```python
from build123d import *

# Parameters (mm, degrees)
BOSS_EXTRUDE1_DEPTH         = 19.05
SKETCH2_R                   = 3.175
CUT_EXTRUDE1_DEPTH          = 42.790767895
CHAMFER1_SIZE               = 3.175
SKETCH3_R                   = 25.2095
BOSS_EXTRUDE2_DEPTH         = 38.1
CHAMFER2_SIZE               = 0.79375
F_4_40_TAPPED_HOLE1_REACH   = 77.334
F_4_40_TAPPED_HOLE1_BORE_R  = 1.1303
F_3_8_16_TAPPED_HOLE1_D     = 7.9375
F_3_8_16_TAPPED_HOLE1_DEPTH = 25.4
F_3_8_16_TAPPED_HOLE1_TIP   = 2.384665582


with BuildPart() as part:
    # Sketch1 → Boss-Extrude1 (new body)
    with BuildSketch(Plane.XY):
        Polygon((-7.14375, 15.875), (-7.14375, -4.7625), (-14.2875, -4.7625), (-14.2875, 23.8125), (14.2875, 23.8125), (14.2875, -4.7625), (7.14375, -4.7625), (7.14375, 15.875), align=None)
    extrude(amount=BOSS_EXTRUDE1_DEPTH)

    # Sketch2 → Cut-Extrude1 (cut, through all)
    with BuildSketch(Plane(origin=(14.2875, 0, 0), x_dir=(0, 0, -1), z_dir=(1, 0, 0))):
        with Locations((-9.525, 0)):
            Circle(SKETCH2_R)
    extrude(amount=-CUT_EXTRUDE1_DEPTH, mode=Mode.SUBTRACT)

    # Chamfer1
    chamfer1_edges = [part.edges().sort_by_distance(p)[0] for p in [
        (10.715625, -4.7625, 19.05),
        (-10.715625, -4.7625, 19.05),
        (-10.715625, -4.7625, 0),
        (10.715625, -4.7625, 0),
    ]]
    chamfer(chamfer1_edges, length=CHAMFER1_SIZE)

    # Sketch3 → Boss-Extrude2 (add)
    with BuildSketch(Plane(origin=(0, 23.8125, 0), x_dir=(1, 0, 0), z_dir=(0, 1, 0))):
        with Locations(Location((0, -9.525, 0), (0, 0, 90))):
            Circle(SKETCH3_R)
    extrude(amount=BOSS_EXTRUDE2_DEPTH)

    # Chamfer2
    chamfer2_edges = [part.edges().sort_by_distance(p)[0] for p in [
        (0, 23.8125, 34.7345),
        (0, 61.9125, 34.7345),
    ]]
    chamfer(chamfer2_edges, length=CHAMFER2_SIZE)

    # #4-40 Tapped Hole1 bore → #4-40 Tapped Hole1 (cut, up to next)
    with BuildSketch(Plane.XY.offset(19.05), mode=Mode.PRIVATE) as f_4_40_tapped_hole1_sk1:
        with Locations((-10.715625, 0)):
            Circle(F_4_40_TAPPED_HOLE1_BORE_R)
    f_4_40_tapped_hole1_tool1 = extrude(f_4_40_tapped_hole1_sk1.sketch, amount=-F_4_40_TAPPED_HOLE1_REACH, mode=Mode.PRIVATE) & part.part
    # #4-40 Tapped Hole1 bore → #4-40 Tapped Hole1 (cut, up to next)
    with BuildSketch(Plane.XY.offset(19.05), mode=Mode.PRIVATE) as f_4_40_tapped_hole1_sk2:
        with Locations((10.715625, 0)):
            Circle(F_4_40_TAPPED_HOLE1_BORE_R)
    f_4_40_tapped_hole1_tool2 = extrude(f_4_40_tapped_hole1_sk2.sketch, amount=-F_4_40_TAPPED_HOLE1_REACH, mode=Mode.PRIVATE) & part.part
    add(f_4_40_tapped_hole1_tool1.solids().sort_by_distance((-10.715625, 0, 19.05))[0], mode=Mode.SUBTRACT)
    add(f_4_40_tapped_hole1_tool2.solids().sort_by_distance((10.715625, 0, 19.05))[0], mode=Mode.SUBTRACT)

    # 3/8-16 Tapped Hole1
    with Locations(Plane(origin=(25.2095, 0, 0), x_dir=(0, 0, -1), z_dir=(1, 0, 0))):
        with Locations((-9.525, 51.1429)):
            Hole(F_3_8_16_TAPPED_HOLE1_D / 2, depth=F_3_8_16_TAPPED_HOLE1_DEPTH)
            with Locations((0, 0, -(F_3_8_16_TAPPED_HOLE1_DEPTH + F_3_8_16_TAPPED_HOLE1_TIP / 2))):  # 118° drill point
                Cone(0, F_3_8_16_TAPPED_HOLE1_D / 2, F_3_8_16_TAPPED_HOLE1_TIP, mode=Mode.SUBTRACT)


solid = part.part
```
Could you check a few things on this model? Use its own coordinates, in mm. A direction names the side the tool comes from. Round coordinates to 2 decimals unless told otherwise and drop trailing zeros. Loops run counter-clockwise (first coordinate to the right, second up) from the corner with the lowest first, then second, coordinate; pieces in that order, holes last. Notation, with made-up numbers: M 88.25,-15.75 L 121.25,-15.75 A14 cw 121.25,-3.75 Z; hole C 63.25,23 d1. An arc over 180 degrees is marked long. Write item = value, one per line.
1. Which directions (+Z, -Z, +X, -X, +Y, -Y) give clear straight access to the entire face, cutting with the end or side of a thin tool? Please do faces 1 (the face through (0, 17, 0)), 2 (the face through (0, 17, 19.05)), 3 (the face through (10.766, 0.954, 6.497)), 4 (the face through (11.76, -0.43, 15.82)), 5 (the face through (14.288, 10, 9)).
Results below:
face_1 = -Z, +X, -X, -Y
face_2 = +Z, +X, -X, -Y
face_3 = +X, -X
face_4 = +Z
face_5 = +Z, -Z, +X, -Y
2. I want a section at D-D, the plane y = 36. Write out the boundary of the cut face in (x, z) (1 decimal).
Results below:
outline = C 0,9.5 d50.4
3. I need wall thicknesses on probe 1 along X at (y, z) = (0, 17.5); probe 2 along Z at (x, y) = (-9.25, 0); probe 3 along X at (y, z) = (17.5, 15.5). Which ranges of each line are inside material? Lowest first, please.
Results below:
probe_1 = -14.29 to -11.85, -9.59 to -7.14, 7.14 to 9.59, 11.85 to 14.29
probe_2 = 0 to 6.35, 12.7 to 19.05
probe_3 = -14.29 to 14.29
4. I want a section at C-C, the plane x = 8. Count the separate pieces of the cut face and the enclosed holes in it, and give its area (3 significant figures).
Results below:
separate_pieces = 1
enclosed_holes = 2
area = 2,270 mm²
5. I want a section at A-A, the plane y = 9.5. Write out the boundary of the cut face in (x, z).
Results below:
outline = M -14.29,0 L -7.14,0 L -7.14,19.05 L -14.29,19.05 Z; M 7.14,0 L 14.29,0 L 14.29,19.05 L 7.14,19.05 Z
6. I want a section at B-B, the plane y = 0. Write out the boundary of the cut face in (x, z), and give its area (3 significant figures).
Results below:
outline = M -14.29,0 L -7.14,0 L -7.14,6.35 L -14.29,6.35 Z; M -14.29,12.7 L -11.85,12.7 L -11.85,19.05 L -14.29,19.05 Z; M -9.59,12.7 L -7.14,12.7 L -7.14,19.05 L -9.59,19.05 Z; M 7.14,0 L 14.29,0 L 14.29,6.35 L 7.14,6.35 Z; M 7.14,12.7 L 9.59,12.7 L 9.59,19.05 L 7.14,19.05 Z; M 11.85,12.7 L 14.29,12.7 L 14.29,19.05 L 11.85,19.05 Z
area = 153 mm²
7. Thinking about a two-plate mould opening in X: for faces 6 (the face through (-17.038, 42.607, 28.105)), 7 (the face through (-2.16, 51.83, 9.61)), 8 (the face through (7.144, 5, 9)), 9 (the face through (-7.144, 6, 9)), which applies, +X half, -X half, draft (parallel to the pull), parting line (faces both ways), or undercut?
Results below:
face_6 = parting line
face_7 = +X half
face_8 = undercut
face_9 = undercut
8. Will these pins go through, and if not, where does the flat tip stop? P1, Ø21, axis at y = 8, z = 5.5, coming from the +X side; P2, Ø12, axis at y = 43, z = 21, coming from the +X side; P3, Ø4, axis at y = 0, z = 9.525, coming from the +X side (3 decimals); P4, Ø1, axis at x = -2, y = 34, coming from the -Z side.
Results below:
P1 = 14.29
P2 = 24.61
P3 = through
P4 = -15.64
